Input: part model. Units: mm. Frame: model coordinates. Face numbers are marked on the shaded views. A direction names the side the tool comes from. Coordinates: 2 decimals unless noted, no trailing zeros. Loops run counter-clockwise (first coordinate to the right, second up) from the corner with the lowest first, then second, coordinate; pieces in that order, holes last. Notation, with made-up numbers: M 61.5,-32 L 81.5,-32 A14 cw 81.5,-11 Z; hole C 43.25,38 d10. An arc over 180 degrees is marked long. Use a Markdown table: item, result. Add a question column.
1. Line query: L1, parallel to Z at x = -7.85, y = 3.1 (3 decimals); L2, parallel to X at y = -7, z = -4; L3, parallel to Y at x = 32.5, z = 34. Output: solid intervals per line, ascending. Write a range as [from, to].
2. Section C-C on x = 12.5. Output: boundary loops of the cut face in (y, z).
3. Section B-B on y = -38. Output: boundary loops of the cut face in (x, z).
4. Section A-A on z = 12. Output: boundary loops of the cut face in (x, y), then the cut area to 3 significant figures.
5. Section D-D on z = 38.5. Output: boundary loops of the cut face in (x, y), then the cut area to 3 significant figures.
6. Set-up query: the marked faces 1, 2 and 3. Return all of +Z, -Z, +X, -X, +Y, -Y with unobstructed straight access to the full face (end or side cutting, diameter ignored); none if empty.
7. Pin query (flat end, axial travel): pin 1 (10 mm diameter, centred on x = 38.5, y = -60.5, fed in from +Z); pin 2 (8 mm diameter, centred on x = 32.5, z = 32.5, fed in from +Y); pin 3 (9 mm diameter, centred on x = 40.5, y = -47.5, fed in from +Z); pin 4 (20 mm diameter, centred on y = -44, z = -4, fed in from -X). Return the tip coordinate at first contact, or that it passes through.
```python
from build123d import *

# Parameters (mm, degrees)
SKETCH1_W                 = 59.5
SKETCH1_H                 = 48
BOSS_EXTRUDE1_DEPTH       = 5
SKETCH2_W                 = 10
SKETCH2_H                 = 48
BOSS_EXTRUDE2_DEPTH       = 72.5
SKETCH3_W                 = 48
SKETCH3_H                 = 10
BOSS_EXTRUDE3_DEPTH       = 30
FILLET1_R                 = 10
F_1_0MM_START             = -72.5
F_1_0MM_DOWEL_SLOT1_DEPTH = 10
FILLET2_R                 = 10
M6_CLEARANCE_HOLE1_D      = 16.15
CHAMFER1_SIZE             = 5
CHAMFER2_SIZE             = 4
SKETCH14_W                = 15
SKETCH14_H                = 5
BOSS_EXTRUDE4_DEPTH       = 20
CHAMFER3_SIZE             = 10
FILLET3_R                 = 2
M2_START                  = -24.5
M2_CLEARANCE_SLOT1_DEPTH  = 5


# Read off the part's stored shape, not the designer's step: Ø1.0mm Dowel Slot1, M2 Clearance Slot1
with BuildPart() as part:
    # Sketch1 → Boss-Extrude1 (new body)
    with BuildSketch(Plane(origin=(0, 0, 0), x_dir=(1, 0, 0), z_dir=(0, 1, 0))):
        with Locations((5.75, 0)):
            Rectangle(SKETCH1_W, SKETCH1_H)
    extrude(amount=BOSS_EXTRUDE1_DEPTH)

    # Sketch2 → Boss-Extrude2 (add)
    with BuildSketch(Plane.XZ):
        with Locations((30.5, 0)):
            Rectangle(SKETCH2_W, SKETCH2_H)
    extrude(amount=BOSS_EXTRUDE2_DEPTH)

    # Sketch3 → Boss-Extrude3 (add)
    with BuildSketch(Plane(origin=(35.5, 0, 0), x_dir=(0, 0, -1), z_dir=(1, 0, 0))):
        with Locations((0, -67.5)):
            Rectangle(SKETCH3_W, SKETCH3_H)
    extrude(amount=BOSS_EXTRUDE3_DEPTH)

    # Fillet1
    fillet1_edges = [part.edges().sort_by_distance(p)[0] for p in [
        (-24, 2.5, -24),
        (-24, 2.5, 24),
    ]]
    fillet(fillet1_edges, radius=FILLET1_R)

    # Ø1.0mm Dowel Slot1 outline → Ø1.0mm Dowel Slot1 (cut)
    with BuildSketch(Plane(origin=(0, 0, 0), x_dir=(1, 0, 0), z_dir=(0, 1, 0)).offset(F_1_0MM_START)):
        with BuildLine():
            Line((53, 14.75), (48, 14.75))
            ThreePointArc((48, 14.75), (45.25, 12), (48, 9.25))
            Line((48, 9.25), (53, 9.25))
            ThreePointArc((53, 9.25), (55.75, 12), (53, 14.75))
        make_face()
        with BuildLine():
            Line((53, -9.25), (48, -9.25))
            ThreePointArc((48, -9.25), (45.25, -12), (48, -14.75))
            Line((48, -14.75), (53, -14.75))
            ThreePointArc((53, -14.75), (55.75, -12), (53, -9.25))
        make_face()
    extrude(amount=F_1_0MM_DOWEL_SLOT1_DEPTH, mode=Mode.SUBTRACT)

    # Fillet2
    fillet2_edges = [part.edges().sort_by_distance(p)[0] for p in [
        (65.5, -67.5, 24),
        (65.5, -67.5, -24),
    ]]
    fillet(fillet2_edges, radius=FILLET2_R)

    # M6 Clearance Hole1 (through all)
    with Locations(Plane(origin=(0, 5, 0), x_dir=(1, 0, 0), z_dir=(0, 1, 0))):
        with Locations((-7.85, 0)):
            Hole(M6_CLEARANCE_HOLE1_D / 2)

    # Chamfer1
    chamfer1_edges = [part.edges().sort_by_distance(p)[0] for p in [
        (25.5, 0, 0),
        (35.5, -62.5, 0),
    ]]
    chamfer(chamfer1_edges, length=CHAMFER1_SIZE)

    # Chamfer2
    chamfer2_edges = [part.edges().sort_by_distance(p)[0] for p in [
        (35.5, 5, 0),
    ]]
    chamfer(chamfer2_edges, length=CHAMFER2_SIZE)

    # Sketch14 → Boss-Extrude4 (add)
    with BuildSketch(Plane.XY.offset(24)):
        with Locations((33, -22)):
            Rectangle(SKETCH14_W, SKETCH14_H)
    extrude(amount=BOSS_EXTRUDE4_DEPTH)

    # Chamfer3
    # the kernel refuses this chamfer: 10 mm, written as the material it adds along each edge
    with BuildSketch(Plane(origin=(35.5, -19.5, 24), x_dir=(-0.027495876610586317, 0, -0.9996219169112968), z_dir=(0, -1, 0))) as chamfer3_piece_1_section:
        Polygon((CHAMFER3_SIZE * 0.999621916911, CHAMFER3_SIZE * 0.0274958766106), (-CHAMFER3_SIZE * 0.0274958766106, CHAMFER3_SIZE * 0.999621916911), (0, 0), align=None)
    chamfer3_piece_1 = extrude(amount=5, mode=Mode.PRIVATE)
    chamfer3_piece_1 = split(chamfer3_piece_1, bisect_by=Plane(origin=(40.5, -22, 20.111111111), z_dir=(-1, 0, 0)), keep=Keep.TOP, mode=Mode.PRIVATE)
    add(chamfer3_piece_1)

    # Fillet3
    fillet3_edges = [part.edges().sort_by_distance(p)[0] for p in [
        (30.5, -24.5, 24),
        (25.5, -22, 44),
        (40.5, -22, 44),
        (35.5, -24.5, 19),
    ]]
    fillet(fillet3_edges, radius=FILLET3_R)

    # M2 Clearance Slot1 outline → M2 Clearance Slot1 (cut)
    with BuildSketch(Plane(origin=(0, 0, 0), x_dir=(1, 0, 0), z_dir=(0, 1, 0)).offset(M2_START)):
        with BuildLine():
            Line((31, -30.2), (36, -30.2))
            ThreePointArc((36, -30.2), (37.2, -29), (36, -27.8))
            Line((36, -27.8), (31, -27.8))
            ThreePointArc((31, -27.8), (29.8, -29), (31, -30.2))
        make_face()
        with BuildLine():
            Line((31, -39.7), (36, -39.7))
            ThreePointArc((36, -39.7), (37.2, -38.5), (36, -37.3))
            Line((36, -37.3), (31, -37.3))
            ThreePointArc((31, -37.3), (29.8, -38.5), (31, -39.7))
        make_face()
    extrude(amount=M2_CLEARANCE_SLOT1_DEPTH, mode=Mode.SUBTRACT)


solid = part.part
```
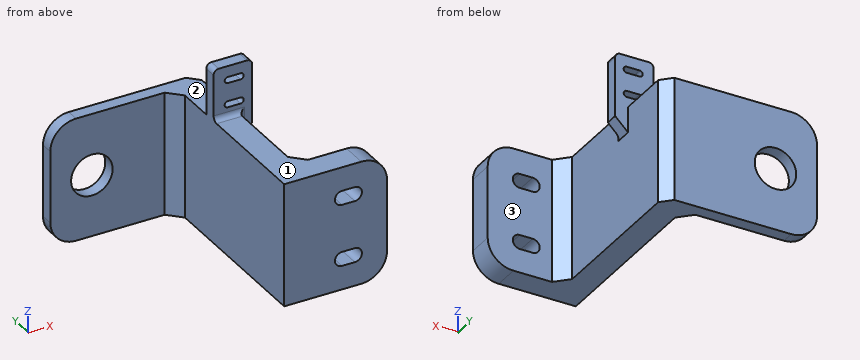
Answers below:
| question | item | result |
|---|---|---|
| 1 | L1 | z = [-24, -8.075], [8.075, 24] |
| 1 | L2 | x = [25.5, 35.5] |
| 1 | L3 | y = [-24.5, -19.5] |
| 2 | outline | M 0,-24 L 5,-24 L 5,24 L 0,24 Z |
| 3 | outline | M 25.5,-24 L 35.5,-24 L 35.5,24 L 25.5,24 Z |
| 4 | outline | M -24,0 L 20.5,0 L 25.5,-5 L 25.5,-72.5 L 45.25,-72.5 L 45.25,-62.5 L 40.5,-62.5 L 35.5,-57.5 L 35.5,1 L 31.5,5 L -24,5 Z; M 55.75,-72.5 L 65.5,-72.5 L 65.5,-62.5 L 55.75,-62.5 Z |
| 4 | area | 1,230 mm² |
| 5 | outline | M 25.5,-24.5 L 29.8,-24.5 L 29.8,-19.5 L 25.5,-19.5 Z; M 37.2,-24.5 L 40.5,-24.5 L 40.5,-19.5 L 37.2,-19.5 Z |
| 5 | area | 38.0 mm² |
| 6 | face 1 | +Z, +X, -X, -Y |
| 6 | face 2 | +Z, +X, -X, +Y |
| 6 | face 3 | +Z, -Z, +X, +Y |
| 7 | pin 1 | stops at z = 24 |
| 7 | pin 2 | stops at y = -19.5 |
| 7 | pin 3 | passes through |
| 7 | pin 4 | stops at x = 25.5 |
